Geometry check sheet. Reference: drawing and pictorial views, mm from the part's lowest x, y, z. A direction names the side the tool comes from. Give positions to 0.01 mm unless a question says otherwise; leave off trailing zeros. Order: outer loops, then holes, each group sorted by start corner. A loop starts at its lowest first (then second) coordinate and runs counter-clockwise, first axis right, second up.
Item 1: Release check for a two-part mould opening along X. For the marked faces 3, 4 and 5 record: released by +X, released by -X, zero draft, split by the parting line, or undercut.
Item 2: Material ranges on line 1 along X through (y, z) = (5, 7.25); line 2 along Z through (x, y) = (3, 1.2); line 3 along Z through (x, y) = (18, 3.25), recorded low to high.
Item 3: Sectioned sample at D-D on x = 3. Record the boundary of the cut face in (y, z), and give its area (3 significant figures).
Item 4: Access from +Z, -Z, +X, -X, +Y, -Y to the whole of each face (thin tool, end or side, straight path). Record for the marked faces 1 and 2.
Item 5: Sectioned sample at B-B on z = 7.5. Record the boundary of the cut face in (x, y), and give its area (3 significant figures).
Item 6: Gauge pin test, flat ends, axial feed: P1, Ø8, axis at x = 31.5, z = 5.5, coming from the +Y side; P2, Ø2, axis at x = 7.5, y = 1.5, coming from the +Z side; P3, Ø4, axis at x = 21.5, y = 7, coming from the +Z side. Record the tip position at first contact, or that the pin passes through.
Item 7: Sectioned sample at A-A on x = 18. Record the boundary of the cut face in (y, z).
Item 8: Sectioned sample at C-C on y = 3.25. Record the boundary of the cut face in (x, z), and give its area (3 significant figures).
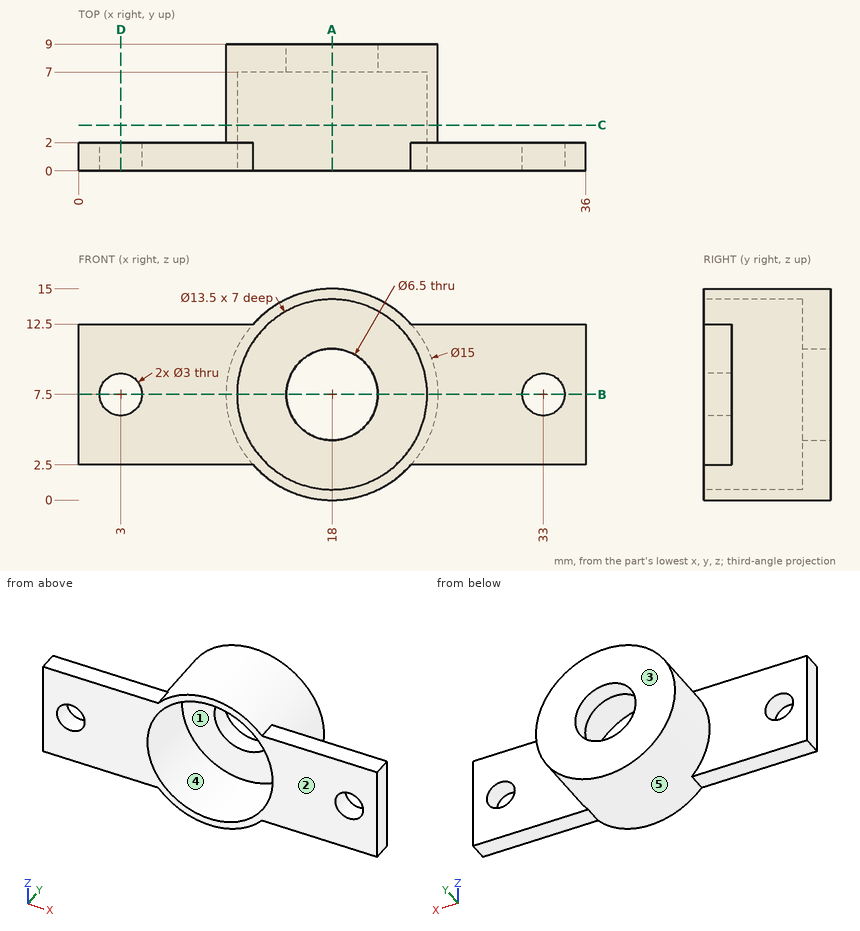
Report:
1. face 3: zero draft
1. face 4: undercut
1. face 5: split by the parting line
2. line 1: x = 10.5 to 11.25, 24.75 to 25.5
2. line 2: z = 2.5 to 6, 9 to 12.5
2. line 3: z = 0 to 0.75, 14.25 to 15
3. outline: (0, 2.5) - (2, 2.5) - (2, 6) - (0, 6) - close; (0, 9) - (2, 9) - (2, 12.5) - (0, 12.5) - close
3. area: 14.0 mm2
4. face 1: -Y
4. face 2: +Z, -Z, +X, -X, -Y
5. outline: (0, 0) - (1.5, 0) - (1.5, 2) - (0, 2) - close; (4.5, 0) - (11.25, 0) - (11.25, 7) - (14.75, 7) - (14.75, 9) - (10.5, 9) - (10.5, 2) - (4.5, 2) - close; (21.25, 7) - (24.75, 7) - (24.75, 0) - (31.5, 0) - (31.5, 2) - (25.5, 2) - (25.5, 9) - (21.25, 9) - close; (34.5, 0) - (36, 0) - (36, 2) - (34.5, 2) - close
5. area: 57.5 mm2
6. P1: stops at y = 2
6. P2: stops at z = 12.5
6. P3: stops at z = 14.85
7. outline: (0, 0) - (9, 0) - (9, 4.25) - (7, 4.25) - (7, 0.75) - (0, 0.75) - close; (0, 14.25) - (7, 14.25) - (7, 10.75) - (9, 10.75) - (9, 15) - (0, 15) - close
8. outline: circle Ø15 at (18, 7.5); hole circle Ø13.5 at (18, 7.5)
8. area: 33.6 mm2
